Autodesk Inventor part; units mm, degrees
ref_plane "YZ Plane" through (0, 0, 0) normal (1, 0, 0) x (0, 1, 0)
ref_plane "XZ Plane" through (0, 0, 0) normal (0, 1, 0) x (-1, 0, 0)
ref_plane "XY Plane" through (0, 0, 0) normal (0, 0, 1) x (1, 0, 0)
sketch "Sketch1" plane through (0, 0, 0) normal (0, 0, 1) x (1, 0, 0)
  circle A0 centre (0, 0) radius 23.8125
  dimension "d0" = 47.625
extrude "Extrusion1" add sketch "Sketch1" along normal blind 20.6375
sketch "Sketch2" plane through (0, 0, 20.6375) normal (0, 0, 1) x (1, 0, 0)
  circle A0 centre (0, 0) radius 23.8125
  circle A1 centre (0, 0) radius 4.7625
  dimension "d3" = 9.525
extrude "Extrusion2" cut sketch "Sketch2" against normal blind 12.7 contours A1
fillet "Fillet1" radius 3.175 2 edges at (-23.8125, 0, 20.6375) (-23.8125, 0, 0)
properties part number "rough pulley"
Verification items for the finished model (mm, model axes). A direction names the side the tool comes from. Give positions to 0.01 mm unless a question says otherwise; leave off trailing zeros. Loops run counter-clockwise (first coordinate to the right, second up) from the corner with the lowest first, then second, coordinate; pieces in that order, holes last.
1. Thickness scan on line 1 (Y direction, x = 0, z = 14.75); line 2 (Z direction, x = -3, y = 1); line 3 (X direction, y = -15.5, z = 5.25). Record the ranges inside material, lowest first.
2. Section check C-C, the plane z = 6. Enter the section's corners in (x, y) (1 decimal), then the cut area to 3 significant figures.
3. Mould release check, pull along Y, two halves, no side actions. Record for faces 1 (the cylindrical face through (-18.897, 14.49, 10.219)), 2 (the cylindrical face through (-3.78, -2.9, 14.38)), 3 (the flat face through (0, 0, 0)): released by +Y, released by -Y, zero draft, split by the parting line, or undercut.
4. Section check D-D, the plane z = 19. Enter the section's corners in (x, y) (1 decimal), then the cut area to 3 significant figures.
5. Go/stop test with flat-tipped pins: pin 1 Ø6 at (x, z) = (-18.5, 12) entering from +Y; pin 2 Ø1.5 at (y, z) = (-17.5, 7.5) entering from -X; pin 3 Ø7.5 at (x, y) = (0, 0) entering from +Z. Record where each tip stops, or that it passes through.
6. Set-up check for faces 4 (the flat face through (0, 0, 7.938)), 5 (the flat face through (0, 5, 20.638)): record each of +Z, -Z, +X, -X, +Y, -Y from which the full face is reachable in a straight line by a thin tool's end or side.
Geometry says:
1. line 1: y = -23.81 to -4.76, 4.76 to 23.81
1. line 2: z = 0 to 7.94
1. line 3: x = -18.08 to 18.08
2. outline: circle Ø47.6 at (0, 0)
2. area: 1,780 mm2
3. face 1: split by the parting line
3. face 2: undercut
3. face 3: zero draft
4. outline: circle Ø46.8 at (0, 0); hole circle Ø9.5 at (0, 0)
4. area: 1,650 mm2
5. pin 1: stops at y = 18.08
5. pin 2: stops at x = -16.93
5. pin 3: stops at z = 7.94
6. face 4: +Z
6. face 5: +Z, +X, -X, +Y, -Y
